```python
from build123d import *

# Parameters (mm, degrees)
F0_W     = 26
F0_H     = 26
F0_R     = 0.85
F0_R_2   = 7.55
F1_DEPTH = 10
F2_R     = 1.5
F3_DEPTH = 26.001


with BuildPart() as f1:
    # F0 (on Top) → F1 (new body)
    with BuildSketch(Plane.XY):
        Rectangle(F0_W, F0_H)
        with Locations((-10, -10)):
            Circle(F0_R, mode=Mode.SUBTRACT)
        with Locations((10, -10)):
            Circle(F0_R, mode=Mode.SUBTRACT)
        with Locations((-10, 10)):
            Circle(F0_R, mode=Mode.SUBTRACT)
        Circle(F0_R_2, mode=Mode.SUBTRACT)
        with Locations((10, 10)):
            Circle(F0_R, mode=Mode.SUBTRACT)
    extrude(amount=F1_DEPTH)

    # F2 (on face) → F3 (cut, through all)
    with BuildSketch(Plane(origin=(-13, 0, 0), x_dir=(0, -1, 0), z_dir=(-1, 0, 0))):
        with Locations((-7, 5)):
            Circle(F2_R)
        with Locations((7, 5)):
            Circle(F2_R)
    extrude(amount=-F3_DEPTH, mode=Mode.SUBTRACT)


solid = f1.part
```
Model file for the job. Use its own axes, mm. Give positions to 0.01 mm unless a question says otherwise; leave off trailing zeros. Loops run counter-clockwise (first coordinate to the right, second up) from the corner with the lowest first, then second, coordinate; pieces in that order, holes last. Notation, with made-up numbers: (-14.75, 83.5) - (-6.75, 83.5) arc R11 cw to (-6.75, 102.5) - close; hole circle Ø9 at (-9, 88.25). An arc over 180 degrees is marked (long way). One line per item, written item: value. Start each with the question number.
1. Slice it at C-C (z = 1). List the corners of the cut face in (x, y).
2. Pull direction Z, two halves, no side cores. Call faces 1 (the cylindrical face through (-0.18, -8.43, 5.45)), 2 (the flat face through (-6, 6, 10)), 3 (the cylindrical face through (-9.543, -9.283, 4.93)): pulls with the +Z half, pulls with the -Z half, needs draft (parallel to the pull), parting line crosses it, or undercut.
3. Slice it at D-D (x = -10). List the corners of the cut face in (y, z).
4. Pin check, flat tip, straight feed: pin 1 (2.5 mm diameter, centred on y = -7, z = 5, fed in from -X). Stop position of the tip, or through.
5. Slice it at B-B (x = -5.75). List the corners of the cut face in (y, z).
6. Slice it at A-A (y = -10). List the corners of the cut face in (x, z), plus the area to 3 significant figures.
7. Probe L1, parallel to Y at x = -10, z = 8.25; L2, parallel to Y at x = -10, z = 4; L3, parallel to X at y = -10.5, z = 2.5. List the from-to ranges inside material, lowest first. Write a range as from..to.
Solution:
1. outline: (-13, -13) - (13, -13) - (13, 13) - (-13, 13) - close; hole circle Ø1.7 at (-10, -10); hole circle Ø1.7 at (-10, 10); hole circle Ø15.1 at (0, 0); hole circle Ø1.7 at (10, -10); hole circle Ø1.7 at (10, 10)
2. face 1: undercut
2. face 2: pulls with the +Z half
2. face 3: needs draft
3. outline: (-13, 0) - (-10.85, 0) - (-10.85, 10) - (-13, 10) - close; (-9.15, 0) - (9.15, 0) - (9.15, 10) - (-9.15, 10) - close; (10.85, 0) - (13, 0) - (13, 10) - (10.85, 10) - close; hole circle Ø3 at (-7, 5); hole circle Ø3 at (7, 5)
4. pin 1: passes through
5. outline: (-13, 0) - (-4.89, 0) - (-4.89, 10) - (-13, 10) - close; (4.89, 0) - (13, 0) - (13, 10) - (4.89, 10) - close; hole circle Ø3 at (-7, 5); hole circle Ø3 at (7, 5)
6. outline: (-13, 0) - (-10.85, 0) - (-10.85, 10) - (-13, 10) - close; (-9.15, 0) - (9.15, 0) - (9.15, 10) - (-9.15, 10) - close; (10.85, 0) - (13, 0) - (13, 10) - (10.85, 10) - close
6. area: 226 mm^2
7. L1: y = -13..-10.85, -9.15..9.15, 10.85..13
7. L2: y = -13..-10.85, -9.15..-8.12, -5.88..5.88, 8.12..9.15, 10.85..13
7. L3: x = -13..-10.69, -9.31..9.31, 10.69..13
